CAD build for the part. Positions are in the model's coordinates, mm. Face numbers are marked on the shaded views. A direction names the side the tool comes from. Round coordinates to 2 decimals unless told otherwise and drop trailing zeros. Order: outer loops, then holes, each group sorted by start corner. A loop starts at its lowest first (then second) coordinate and runs counter-clockwise, first axis right, second up. Notation, with made-up numbers: M -24.75,72.25 L -17.75,72.25 A19 cw -17.75,85.25 Z; hole C 71,-2 d1. An arc over 180 degrees is marked long. Put each result on its own line as item: value.
```python
from build123d import *

# Parameters (mm, degrees)
F1_DEPTH = 50
F2_R     = 7.1
F3_R     = 3.5
F4_DEPTH = 25
F5_R     = 2
F5_R_2   = 8
F6_DEPTH = 25


with BuildPart() as f1:
    # F0 (on Front) → F1 (new body, symmetric)
    with BuildSketch(Plane.XZ):
        with BuildLine():
            ThreePointArc((-13.5, 0), (-9.545942, 9.545942), (0, 13.5))
            Line((0, 13.5), (0, 21.172315))
            ThreePointArc((0, 21.172315), (-14.971087, 14.971087), (-21.172315, 0))
            Line((-21.172315, 0), (-21.172315, -28.827685))
            Line((-21.172315, -28.827685), (-13.5, -28.827685))
            Line((-13.5, -28.827685), (-13.5, 0))
        make_face()
        with BuildLine():
            ThreePointArc((0, 13.5), (9.545942, 9.545942), (13.5, 0))
            Line((13.5, 0), (13.5, -28.827685))
            Line((13.5, -28.827685), (21.172315, -28.827685))
            Line((21.172315, -28.827685), (21.172315, 0))
            ThreePointArc((21.172315, 0), (14.971087, 14.971087), (0, 21.172315))
            Line((0, 21.172315), (0, 13.5))
        make_face()
    extrude(amount=F1_DEPTH, both=True)

    # F2
    f2_edges = [f1.edges().sort_by_distance(p)[0] for p in [
        (17.336157, 50, -28.827685),
        (-17.336157, 50, -28.827685),
        (-17.336157, -50, -28.827685),
        (17.336157, -50, -28.827685),
    ]]
    fillet(f2_edges, radius=F2_R)

    # F3 (on Right) → F4 (cut, symmetric)
    with BuildSketch(Plane.YZ):
        with Locations((-43.000714, -21.827685)):
            Circle(F3_R)
    extrude(amount=F4_DEPTH, both=True, mode=Mode.SUBTRACT)

    # F5 (on Top) → F6 (cut)
    with BuildSketch(Plane.XY):
        with Locations((0, -13)):
            Circle(F5_R)
        with Locations((0, 12)):
            Circle(F5_R_2)
    extrude(amount=F6_DEPTH, mode=Mode.SUBTRACT)


solid = f1.part
```
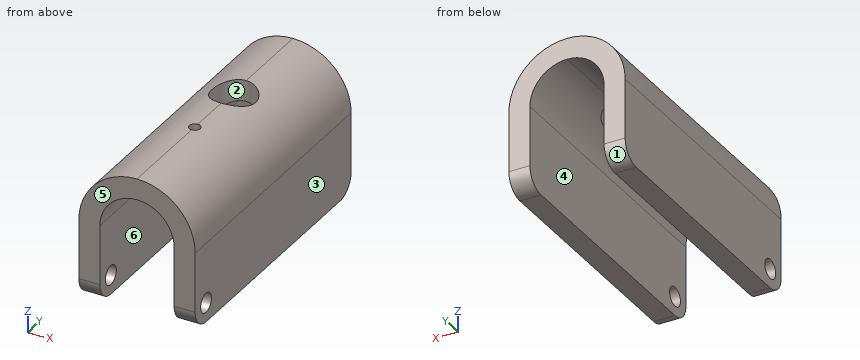
Item 1: Band-saw the part on B-B on y = 6.5. Give the cut face in (x, z), and give its area (3 significant figures).
Answers below:
outline: M -21.17,-28.83 L -13.5,-28.83 L -13.5,0 A13.5 cw -5.81,12.19 L -5.81,20.36 A21.17 ccw -21.17,0 Z; M 5.81,12.19 A13.5 cw 13.5,0 L 13.5,-28.83 L 21.17,-28.83 L 21.17,0 A21.17 ccw 5.81,20.36 Z
area: 769 mm²
Item 2: Mould opens along X. For the marked faces 1, 2, 3 and 4 say: pulls with the +X half, pulls with the -X half, needs draft (parallel to the pull), parting line crosses it, or undercut.
Answers below:
face 1: needs draft
face 2: undercut
face 3: pulls with the +X half
face 4: undercut
Item 3: Pin check, flat tips, straight feed: P1, Ø10, axis at y = -14.5, z = 11.5, coming from the -X side; P2, Ø6, axis at x = 5, y = 39.5, coming from the -Z side; P3, Ø2, axis at x = 3.5, y = 34.5, coming from the +Z side; P4, Ø9.5, axis at x = 0, y = 12, coming from the +Z side. Stop position of each tip, or through.
Answers below:
P1: x = -20.15
P2: z = 10.87
P3: z = 21.02
P4: through
Item 4: Tool access for the marked faces 5 and 6: list every direction of +Z, -Z, +X, -X, +Y, -Y with a clear straight run to the whole face (end or side of a thin tool).
Answers below:
face 5: +Z, -Z, +X, -X, -Y
face 6: -Z, +Y, -Y
Item 5: Band-saw the part on C-C on x = -17.5. Give the cut face in (y, z).
Answers below:
outline: M -50,-21.73 A7.1 ccw -42.9,-28.83 L 42.9,-28.83 A7.1 ccw 50,-21.73 L 50,11.92 L -50,11.92 Z; hole C -43,-21.83 d7
Item 6: Band-saw the part on A-A on z = -9. Give the cut face in (x, y).
Answers below:
outline: M -21.17,-50 L -13.5,-50 L -13.5,50 L -21.17,50 Z; M 13.5,-50 L 21.17,-50 L 21.17,50 L 13.5,50 Z
Item 7: Band-saw the part on D-D on y = -20. Give the cut face in (x, z).
Answers below:
outline: M -21.17,-28.83 L -13.5,-28.83 L -13.5,0 A13.5 cw 0,13.5 A13.5 cw 13.5,0 L 13.5,-28.83 L 21.17,-28.83 L 21.17,0 A21.17 ccw 0,21.17 A21.17 ccw -21.17,0 Z
Item 8: Probe line 1 along Y through (x, z) = (0, 16); line 2 along X through (y, z) = (-33.5, -19.5); line 3 along Z through (x, y) = (19.5, -43). List the from-to ranges inside material, lowest first. Write a range as [from, to].
Answers below:
line 1: [-50, -15], [-11, 4], [20, 50]
line 2: [-21.17, -13.5], [13.5, 21.17]
line 3: [-28.83, -25.33], [-18.33, 8.25]
